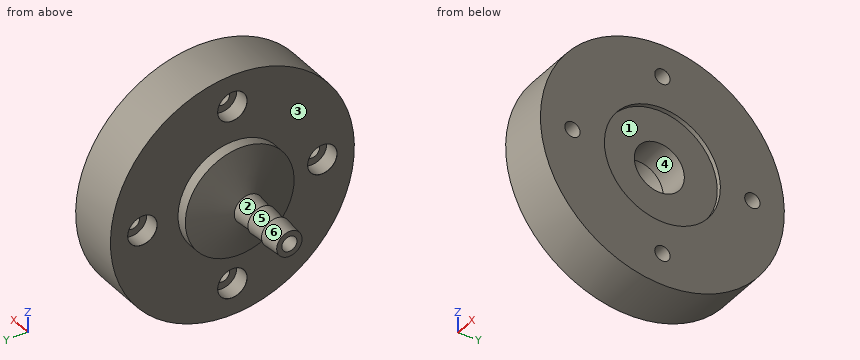
```python
from build123d import *

# Parameters (mm, degrees)
CBORE_FOR_M3_HEX_SOCKET_HEAD_CAP_SCR_2_COUNT = 2
CBORE_FOR_M3_HEX_SOCKET_HEAD_CAP_SCR_2_PITCH = 28.243387552
CBORE_FOR_M3_HEX_SOCKET_HEAD_CAP_SCR_3_COUNT = 2
CBORE_FOR_M3_HEX_SOCKET_HEAD_CAP_SCR_3_PITCH = 39.942181723
CBORE_FOR_M3_HEX_SOCKET_HEAD_CAP_SCR_4_COUNT = 2
CBORE_FOR_M3_HEX_SOCKET_HEAD_CAP_SCR_4_PITCH = 28.243387552


with BuildPart() as part:
    # Sketch1 → Revolve17 (revolve)
    with BuildSketch(Plane.XY, mode=Mode.PRIVATE) as revolve17_sk:
        Polygon((-71.291859268, 14.884170222), (-71.291859268, 14.534170222), (-66.841859268, 14.884170222), (-66.841859268, 14.534170222), (-62.371609448, 14.884170222), (-62.371609448, 14.534170222), (-59.488918076, 23.788045652), (-57.091214807, 23.788045652), (-57.091214807, 38.788045652), (-45.705811648, 38.788045652), (-45.705811648, 26.202485582), (-45.705811648, 24.589170222), (-46.715811648, 24.589170222), (-46.715811648, 17.270420222), (-53.637545484, 17.270420222), (-59.488918076, 13.399170222), (-75.741859268, 13.399170222), (-75.741859268, 14.534170222), align=None)
    revolve(revolve17_sk.sketch.rotate(Axis((-795.163849313, 11.714170222, 0), (1, 0, 0)), 90), axis=Axis((-795.163849313, 11.714170222, 0), (1, 0, 0)))

    # Sketch4 → CBORE for M3 Hex Socket Head Cap Screw1 (revolve, cut)
    with BuildSketch(Plane(origin=(-57.091214807, 11.714170222, -19.971090862), x_dir=(0, 0, 1), z_dir=(0, 1, 0))):
        Polygon((0, 0), (0, 11.385403159), (1.7, 11.385403159), (1.7, 3.4), (3.25, 3.4), (3.25, 0.025), (3.275, 0), align=None)
    cbore_for_m3_hex_socket_head_cap_screw1 = revolve(axis=Axis((-63.441214807, 11.714170222, -19.971090862), (1, 0, 0)), mode=Mode.SUBTRACT)

    # CBORE for M3 Hex Socket Head Cap Scr 2: CBORE for M3 Hex Socket Head Cap Screw1 ×2
    with Locations(*[Vector(0, 0.7071067811865475, 0.7071067811865476) * (i * CBORE_FOR_M3_HEX_SOCKET_HEAD_CAP_SCR_2_PITCH) for i in range(1, CBORE_FOR_M3_HEX_SOCKET_HEAD_CAP_SCR_2_COUNT)]):
        add(cbore_for_m3_hex_socket_head_cap_screw1, mode=Mode.SUBTRACT)

    # CBORE for M3 Hex Socket Head Cap Scr 3: CBORE for M3 Hex Socket Head Cap Screw1 ×2
    with Locations(*[(0, 0, i * CBORE_FOR_M3_HEX_SOCKET_HEAD_CAP_SCR_3_PITCH) for i in range(1, CBORE_FOR_M3_HEX_SOCKET_HEAD_CAP_SCR_3_COUNT)]):
        add(cbore_for_m3_hex_socket_head_cap_screw1, mode=Mode.SUBTRACT)

    # CBORE for M3 Hex Socket Head Cap Scr 4: CBORE for M3 Hex Socket Head Cap Screw1 ×2
    with Locations(*[Vector(0, -0.7071067811865476, 0.7071067811865475) * (i * CBORE_FOR_M3_HEX_SOCKET_HEAD_CAP_SCR_4_PITCH) for i in range(1, CBORE_FOR_M3_HEX_SOCKET_HEAD_CAP_SCR_4_COUNT)]):
        add(cbore_for_m3_hex_socket_head_cap_screw1, mode=Mode.SUBTRACT)


solid = part.part
```
Geometry: final body of the model. Coordinates: model frame, mm. Face numbers are marked on the shaded views. A direction names the side the tool comes from. Round coordinates to 2 decimals unless told otherwise and drop trailing zeros. Write each loop counter-clockwise with the first axis right and the second up, starting at its lowest first coordinate (ties: lowest second). Pieces come first, ordered by that corner, then holes.
Item 1: Section query C-C (y = -3). Return loops of the section in (x, z), plus the area to 3 significant figures.
Item 2: Material intervals for L1, parallel to Y at x = -51.25, z = 0; L2, parallel to X at y = -4, z = -13.5; L3, parallel to Z at x = -57, y = 30.5, sorted ascending.
Item 3: Section query B-B (x = -65). Return loops of the section in (y, z) (3 decimals).
Item 4: Section query A-A (z = 0). Give the number of separate pieces and of enclosed holes in the cut face, plus the area to 3 significant figures.
Item 5: Mould query, pull axis Y, two halves, no side actions, for the marked faces 1, 2 and 3. Classes: +Y half, -Y half, draft (parallel to the pull), parting line (faces both ways), or undercut.
Item 6: Pin query (flat end, axial travel): P1, Ø5, axis at x = -72.5, y = 18, coming from the +Z side; P2, Ø1, axis at x = -72, y = 14.5, coming from the +Z side; P3, Ø1, axis at x = -53.5, y = -5.5, coming from the -Z side; P4, Ø5, axis at x = -58.5, y = 6.5, coming from the -Z side. Return the tip coordinate at first contact, or that it passes through.
Item 7: Section query D-D (z = -15.5). Return loops of the section in (x, y), plus the area to 3 significant figures.
Item 8: Set-up query: the marked faces 4, 5 and 6. Return all of +Z, -Z, +X, -X, +Y, -Y with unobstructed straight access to the full face (end or side cutting, diameter ignored); none if empty.
Completed:
1. outline: (-57.09, -22.73) - (-45.71, -22.73) - (-45.71, 22.73) - (-57.09, 22.73) - close
1. area: 517 mm2
2. L1: y = -15.36 to -9.96, -6.56 to 6.16, 17.27 to 29.99, 33.39 to 38.79
2. L2: x = -57.09 to -45.71
2. L3: z = -19.5 to -3.03, 3.03 to 19.5
3. outline: circle Ø5.928 at (11.714, 0); hole circle Ø3.37 at (11.714, 0)
4. separate pieces: 4
4. enclosed holes: 0
4. area: 499 mm2
5. face 1: undercut
5. face 2: parting line
5. face 3: draft
6. P1: passes through
6. P2: stops at z = 2.12
6. P3: stops at z = -21.3
6. P4: stops at z = -26.89
7. outline: (-57.09, -10.48) - (-45.71, -10.48) - (-45.71, 33.91) - (-57.09, 33.91) - close
7. area: 505 mm2
8. face 4: +X
8. face 5: none
8. face 6: -X
